Part model, mm, in its own coordinate system. A direction names the side the tool comes from. Round coordinates to 2 decimals unless told otherwise and drop trailing zeros. Order: outer loops, then holes, each group sorted by start corner. A loop starts at its lowest first (then second) coordinate and runs counter-clockwise, first axis right, second up. Notation, with made-up numbers: (-39, 44) - (-32, 44) arc R28 ccw to (-32, 73) - close; hole circle Ø2 at (61, -28). An arc over 180 degrees is marked (long way). Answer as a JSON object with one key per item and string values.
```python
from build123d import *

# Parameters (mm, degrees)
F1_DEPTH = 19.05
F3_DEPTH = 25.4
F4_W     = 88.9
F4_H     = 19.05
F4_W_2   = 38.1
F4_H_2   = 44.45
F5_DEPTH = 19.05
F6_DEPTH = 25.4


with BuildPart() as f1:
    # F0 (on Front) → F1 (new body)
    with BuildSketch(Plane.XZ):
        with BuildLine():
            Line((754.4526390882, -127), (1219.7509574175, -127))
            Line((1219.7509574175, -127), (1218.1324014764, 0.3078377019))
            ThreePointArc((1218.1324014764, 0.3078377019), (971.9574719259, -30.9690211882), (754.4526390882, 88.4963944497))
            Line((754.4526390882, 88.4963944497), (754.4526390882, -127))
        make_face()
        with BuildLine():
            Line((152.9509574175, -127), (754.4526390882, -127))
            Line((754.4526390882, -127), (754.4526390882, 88.4963944497))
            ThreePointArc((754.4526390882, 88.4963944497), (389.4863986152, 159.9886479518), (152.9509574175, -127))
        make_face()
    extrude(amount=F1_DEPTH)

    # F2 (on face) → F3 (cut)
    with BuildSketch(Plane.XZ.offset(19.05)):
        Polygon((349.2892183732, -69.85), (250.3213995681, 41.6179700068), (186.5879998116, -69.85), (250.3213995681, -69.85), (313.393828538, -69.85), (314.0547993247, -69.85), align=None)
        Polygon((398.7721789756, 33.9153755605), (456.7740343957, 116.6469860451), (488.14527835, 161.3937189979), (263.1718880821, 55.8370334618), (275.3515595595, 42.1190060128), (321.7644516922, -10.1560762376), (345.300821131, -36.6652117763), (347.0743577182, -38.6627552758), (347.5783524621, -39.1055249546), (349.2892183732, -36.6652117763), align=None)
        Polygon((511.9904369348, 162.2207457014), (368.3392183732, -69.85), (655.6416554964, -69.85), align=None)
        Polygon((535.8355955196, 161.3937189979), (558.164750711, 129.544272866), (618.0461857734, 44.1317024412), (675.8040291483, -38.2518586693), (682.4792207708, -32.3878542947), (696.5108706698, -16.5849944314), (738.8565177121, 31.1059279369), (760.8124771809, 55.8333800289), align=None)
        Polygon((837.3928740579, -69.85), (773.6627312413, 41.6141579413), (674.6916554964, -69.85), align=None)
    extrude(amount=-F3_DEPTH, mode=Mode.SUBTRACT)

    # F4 (on face) → F5 (join)
    with BuildSketch(Plane.XZ.offset(19.05)):
        with Locations((705.4009574175, -136.525)):
            Rectangle(F4_W, F4_H)
        with Locations((489.5009574175, -136.525)):
            Rectangle(F4_W, F4_H)
        Polygon((250.3213995681, -127), (229.1509574175, -127), (229.1509574175, -146.05), (318.0509574175, -146.05), (318.0509574175, -127), align=None)
        Polygon((583.8160462156, -69.85), (655.6416554964, -69.85), (583.8160462156, 46.1853728507), align=None)
        Polygon((583.8160462156, -69.85), (583.8160462156, 46.1853728507), (550.0904369348, 100.6696116438), (550.0904369348, -69.85), align=None)
        Polygon((550.0904369348, 100.6696116438), (583.8160462156, 46.1853728507), (583.8160462156, 92.9562538667), (578.4083301084, 100.6696116438), align=None)
        Polygon((550.0904369348, -69.85), (550.0904369348, 100.6696116438), (541.6532601983, 114.3), (511.9904369348, 114.3), (511.9904369348, -69.85), align=None)
        Polygon((541.6532601983, 114.3), (550.0904369348, 100.6696116438), (550.0904369348, 114.3), align=None)
        Polygon((578.4083301084, 100.6696116438), (583.8160462156, 92.9562538667), (618.0461857734, 44.1317024412), (675.8040291483, -38.2518586693), (682.4792207708, -32.3878542947), (696.5108706698, -16.5849944314), (738.8565177121, 31.1059279369), (760.8124771809, 55.8333800289), (535.8355955196, 161.3937189979), (558.164750711, 129.544272866), align=None)
        with Locations((531.0404369348, -92.075)):
            Rectangle(F4_W_2, F4_H_2)
        Polygon((511.9904369348, 114.3), (541.6532601983, 114.3), (511.9904369348, 162.2207457014), (482.3276136712, 114.3), align=None)
        with Locations((492.9404369348, -92.075)):
            Rectangle(F4_W_2, F4_H_2)
        Polygon((473.8904369348, -69.85), (511.9904369348, -69.85), (511.9904369348, 114.3), (482.3276136712, 114.3), (473.8904369348, 100.6696116438), align=None)
        Polygon((440.164827654, -69.85), (473.8904369348, -69.85), (473.8904369348, 100.6696116438), (440.164827654, 46.1853728507), align=None)
        Polygon((473.8904369348, 100.6696116438), (482.3276136712, 114.3), (473.8904369348, 114.3), align=None)
        Polygon((368.3392183732, -69.85), (440.164827654, -69.85), (440.164827654, 46.1853728507), align=None)
        Polygon((440.164827654, 46.1853728507), (473.8904369348, 100.6696116438), (445.5725437612, 100.6696116438), (440.164827654, 92.9562538667), align=None)
    extrude(amount=-F5_DEPTH)

    # F4 (on face) → F6 (cut)
    with BuildSketch(Plane.XZ.offset(19.05)):
        Polygon((583.8160462156, -69.85), (655.6416554964, -69.85), (583.8160462156, 46.1853728507), align=None)
        Polygon((550.0904369348, -69.85), (550.0904369348, 100.6696116438), (541.6532601983, 114.3), (511.9904369348, 114.3), (511.9904369348, -69.85), align=None)
        Polygon((541.6532601983, 114.3), (550.0904369348, 100.6696116438), (550.0904369348, 114.3), align=None)
        Polygon((578.4083301084, 100.6696116438), (583.8160462156, 92.9562538667), (618.0461857734, 44.1317024412), (675.8040291483, -38.2518586693), (682.4792207708, -32.3878542947), (696.5108706698, -16.5849944314), (738.8565177121, 31.1059279369), (760.8124771809, 55.8333800289), (535.8355955196, 161.3937189979), (558.164750711, 129.544272866), align=None)
        with Locations((531.0404369348, -92.075)):
            Rectangle(F4_W_2, F4_H_2)
        with Locations((492.9404369348, -92.075)):
            Rectangle(F4_W_2, F4_H_2)
        Polygon((473.8904369348, -69.85), (511.9904369348, -69.85), (511.9904369348, 114.3), (482.3276136712, 114.3), (473.8904369348, 100.6696116438), align=None)
        Polygon((473.8904369348, 100.6696116438), (482.3276136712, 114.3), (473.8904369348, 114.3), align=None)
        Polygon((368.3392183732, -69.85), (440.164827654, -69.85), (440.164827654, 46.1853728507), align=None)
    extrude(amount=-F6_DEPTH, mode=Mode.SUBTRACT)


solid = f1.part
```
Item 1: Drop flat-ended pins along their axis: P1, Ø5.5, axis at y = -12.5, z = -38, coming from the +X side; P2, Ø5.5, axis at y = -5.5, z = -137, coming from the -X side; P3, Ø5, axis at y = -5, z = -78.5, coming from the +X side; P4, Ø8, axis at x = 628, z = 38, coming from the -Y side. Give the stop position or say it passes through.
Taken from the geometry:
{"P1": "x = 1218.65", "P2": "x = 229.15", "P3": "x = 1219.17", "P4": "through"}
Item 2: Cut at D-D (y = -11). State how many separate pieces and enclosed holes the cut face has, plus the area to 3 significant figures.
Taken from the geometry:
{"separate pieces": "1", "enclosed holes": "7", "area": "137,000 mm2"}
Item 3: Cut at C-C (z = -86.5). Write the cut outline in (x, y).
Taken from the geometry:
{"outline": "(161.54, -19.05) - (473.89, -19.05) - (473.89, 0) - (161.54, 0) - close; (550.09, -19.05) - (1219.24, -19.05) - (1219.24, 0) - (550.09, 0) - close"}
Item 4: Cut at A-A (z = 76.5). Write the cut outline in (x, y), plus the area to 3 significant figures.
Taken from the geometry:
{"outline": "(256.78, -19.05) - (307.21, -19.05) - (307.21, 0) - (256.78, 0) - close; (428.63, -19.05) - (473.89, -19.05) - (473.89, 0) - (428.63, 0) - close; (550.09, -19.05) - (595.35, -19.05) - (595.35, 0) - (550.09, 0) - close; (716.77, -19.05) - (766.21, -19.05) - (766.21, 0) - (716.77, 0) - close", "area": "3,630 mm2"}
Item 5: Two-plate mould, pull along Z, no slides. Class faces 4 (the flat face through (489, -10, -146.05)), 5 (the flat face through (679, -19.05, -53)), 6 (the flat face through (440.165, -10, -13)): pulls with the +Z half, pulls with the -Z half, needs draft (parallel to the pull), parting line crosses it, or undercut.
Taken from the geometry:
{"face 4": "pulls with the -Z half", "face 5": "needs draft", "face 6": "undercut"}
Item 6: Probe L1, parallel to Z at x = 746.5, y = -9; L2, parallel to X at y = -17.25, z = -65; L3, parallel to X at y = -8, z = -67. List the from-to ranges inside material, lowest first. Write a range as from..to.
Taken from the geometry:
{"L1": "-146.05..-69.85, 11.02..39.71, 62.55..95.42", "L2": "168.11..189.36, 344.98..371.34, 440.16..473.89, 550.09..583.82, 652.64..679, 834.62..1218.96", "L3": "167.44..188.22, 346.76..370.1, 440.16..473.89, 550.09..583.82, 653.88..677.22, 835.76..1218.99"}
Item 7: Cut at B-B (x = 500). Write the cut outline in (y, z), plus the area to 3 significant figures.
Taken from the geometry:
{"outline": "(-19.05, -146.05) - (0, -146.05) - (0, -114.3) - (-19.05, -114.3) - close; (-19.05, 114.3) - (0, 114.3) - (0, 181.07) - (-19.05, 181.07) - close", "area": "1,880 mm2"}
Item 8: Tool access for faces 1 (the flat face through (550.09, -10, -2)), 2 (the flat face through (597, -9, -127)), 3 (the flat face through (191, -9, -127)): list every direction of +Z, -Z, +X, -X, +Y, -Y with a clear straight run to the whole face (end or side of a thin tool).
Taken from the geometry:
{"face 1": "+Y, -Y", "face 2": "-Z, +Y, -Y", "face 3": "-Z, -X, +Y, -Y"}
